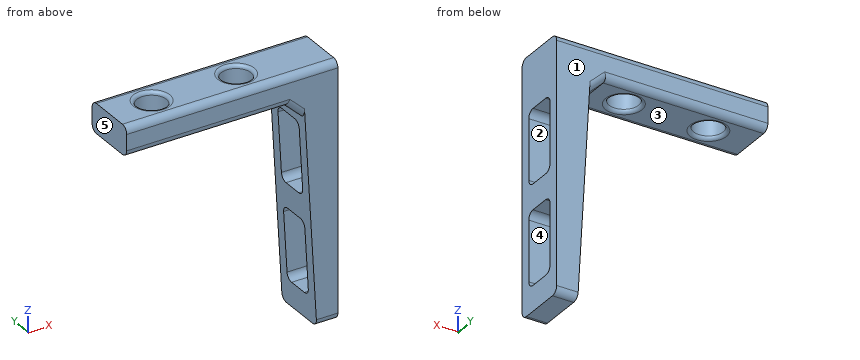
Autodesk Inventor part; units mm, degrees
ref_plane "YZ Plane" through (0, 0, 0) normal (1, 0, 0) x (0, 1, 0)
ref_plane "XZ Plane" through (0, 0, 0) normal (0, 1, 0) x (-1, 0, 0)
ref_plane "XY Plane" through (0, 0, 0) normal (0, 0, 1) x (1, 0, 0)
sketch "Szkic1" plane through (0, 0, 0) normal (0, 1, 0) x (-1, 0, 0)
  line L0 (0, 0) -> (25, 0)
  line L1 (25, 0) -> (25, -3.5)
  line L2 (25, -3.5) -> (4, -3.5)
  line L3 (4, -3.5) -> (2.5, -30)
  line L4 (2.5, -30) -> (0, -30)
  line L5 (0, -30) -> (0, 0)
  dimension "d0" = 25
  dimension "d1" = 30
  dimension "d2" = 3.5
  dimension "d3" = 2.5
  dimension "d4" = 4
extrude "Wyciągnięcie proste1" add sketch "Szkic1" along normal blind 6.5
sketch "Szkic2" plane through (0, 0, 0) normal (1, 0, 0) x (0, 0, -1)
  line L0 (0, 0) -> (30, 0)
  line L1 (30, 0) -> (30, 6.5)
  line L2 (0, 6.5) -> (30, 6.5)
  line L3 (0, 0) -> (0, 6.5)
  line L4 (30, 3.25) -> (0, 3.25) construction
  line L5 (18.25, 5.25) -> (27, 5.25)
  line L6 (27, 5.25) -> (27, 1.25)
  line L7 (27, 1.25) -> (18.25, 1.25)
  line L8 (18.25, 1.25) -> (18.25, 5.25)
  line L9 (18.25, 5.25) -> (27, 1.25) construction
  line L10 (27, 5.25) -> (18.25, 1.25) construction
  line L11 (6.5, 5.25) -> (15.25, 5.25)
  line L12 (15.25, 5.25) -> (15.25, 1.25)
  line L13 (15.25, 1.25) -> (6.5, 1.25)
  line L14 (6.5, 1.25) -> (6.5, 5.25)
  line L15 (6.5, 5.25) -> (15.25, 1.25) construction
  line L16 (15.25, 5.25) -> (6.5, 1.25) construction
  line L17 (3.5, 0) -> (3.5, 6.5)
  point P0 (22.625, 3.25)
  point P1 (10.875, 3.25)
  dimension "d7" = 26.5
  dimension "d8" = 3
  dimension "d9" = 3
  dimension "d10" = 3
  dimension "d11" = 4
extrude "Wyciągnięcie proste2" cut sketch "Szkic2" against normal up to surface contours L5 L6 L7 L8 | L11 L12 L13 L14 surface through (-2.5, 0, -30) normal (-0.9984018, 0, -0.0565133)
sketch "Szkic3" plane through (-25, 0, 0) normal (0, 0, 1) x (1, 0, 0)
  line L0 (0, 0) -> (25, 0)
  line L1 (25, 0) -> (25, 6.5)
  line L2 (0, 6.5) -> (25, 6.5) construction
  line L3 (0, 0) -> (0, 6.5)
  line L4 (0, 3.25) -> (25, 3.25) construction
  circle A0 centre (15, 3.25) radius 1.75
  circle A1 centre (5, 3.25) radius 1.75
  dimension "d14" = 3.5
  dimension "d15" = 10
  dimension "d16" = 10
extrude "Wyciągnięcie proste3" cut sketch "Szkic3" against normal up to surface (3.5 mm away)
chamfer "Faza1" distance 2 angle 45 1 edges at (-4, 3.25, -3.5)
fillet "Zaokrąglenie1" radius 0.8 16 edges at (-1.25, 6.5, -30) (-1.25, 0, -30) (-12.5, 6.5, 0) (-12.5, 0, 0) (-15.5, 0, -3.5) (-15.5, 6.5, -3.5) (-4.9435, 6.5, -4.4984) (-4.9435, 0, -4.4984) (-1.3349, 5.25, -27) (-1.5825, 5.25, -18.25) (-1.3349, 1.25, -27) (-1.5825, 1.25, -18.25) (-1.6675, 5.25, -15.25) (-1.6675, 1.25, -15.25) (-1.9151, 1.25, -6.5) (-1.9151, 5.25, -6.5)
fillet "Zaokrąglenie2" radius 0.4 4 edges at (-11.75, 3.25, -3.5) (-21.75, 3.25, -3.5) (-11.75, 3.25, 0) (-21.75, 3.25, 0)
equation "\"d9\" = d8"
properties part number "noga1"
Input: part model. Units: mm. Frame: model coordinates. Face numbers are marked on the shaded views. A direction names the side the tool comes from. Give positions to 0.01 mm unless a question says otherwise; leave off trailing zeros. Write each loop counter-clockwise with the first axis right and the second up, starting at its lowest first coordinate (ties: lowest second). Pieces come first, ordered by that corner, then holes. Notation, with made-up numbers: M -9.5,-3 L 23.5,-3 A20 cw 23.5,25 Z; hole C -17,-20 d7. An arc over 180 degrees is marked long. Use one line per item in the form item = value.
1. First-contact query: P1, Ø3, axis at y = 1.5, z = -20, coming from the -X side; P2, Ø1, axis at x = -21.5, y = 5.5, coming from the +Z side; P3, Ø2, axis at x = -19.5, y = 4, coming from the -Z side. Flat tips, straight axial feed; report the tip coordinate or a pass-through.
Outcome:
P1 = -3.15
P2 = 0
P3 = -3.41
2. Mould query, pull axis Z, two halves, no side actions, for the marked faces 3, 4 and 5. Classes: released by +Z, released by -Z, zero draft, split by the parting line, or undercut.
Outcome:
face_3 = released by -Z
face_4 = undercut
face_5 = zero draft
3. Cut plane A-A on x = -20. Return loops of the section in (y, z).
Outcome:
outline = M 0,-2.7 A0.8 ccw 0.8,-3.5 L 1.1,-3.5 A0.4 ccw 1.5,-3.1 L 1.5,-0.4 A0.4 ccw 1.1,0 L 0.8,0 A0.8 ccw 0,-0.8 Z; M 5,-3.1 A0.4 ccw 5.4,-3.5 L 5.7,-3.5 A0.8 ccw 6.5,-2.7 L 6.5,-0.8 A0.8 ccw 5.7,0 L 5.4,0 A0.4 ccw 5,-0.4 Z
4. Reachability of the marked faces 1 and 2 from +Z, -Z, +X, -X, +Y, -Y: full face, straight path, thin tool, end or side. Return the list, or none.
Outcome:
face_1 = +Z, -Z, +X, -X, +Y
face_2 = +X, -X
5. Ray query, L1, parallel to Z at x = -2, y = 3.5; L2, parallel to Y at x = -20, z = -2.1; L3, parallel to Z at x = -3, y = 2. Return the intervals inside material, ascending.
Outcome:
L1 = -30 to -27, -18.25 to -15.25, -6.5 to 0
L2 = 0 to 1.5, 5 to 6.5
L3 = -18.25 to -15.25, -6.5 to 0
6. Cut plane C-C on x = -2. Return loops of the section in (y, z).
Outcome:
outline = M 0,-29.2 A0.8 ccw 0.8,-30 L 5.7,-30 A0.8 ccw 6.5,-29.2 L 6.5,-0.8 A0.8 ccw 5.7,0 L 0.8,0 A0.8 ccw 0,-0.8 Z; hole M 1.25,-26.2 A0.8 ccw 2.05,-27 L 4.45,-27 A0.8 ccw 5.25,-26.2 L 5.25,-19.05 A0.8 ccw 4.45,-18.25 L 2.05,-18.25 A0.8 ccw 1.25,-19.05 Z; hole M 1.25,-14.45 A0.8 ccw 2.05,-15.25 L 4.45,-15.25 A0.8 ccw 5.25,-14.45 L 5.25,-7.3 A0.8 ccw 4.45,-6.5 L 2.05,-6.5 A0.8 ccw 1.25,-7.3 Z
7. Cut plane B-B on y = 3.25. State how many separate pieces and enclosed holes the cut face has, and give its area (3 significant figures).
Outcome:
separate_pieces = 5
enclosed_holes = 0
area = 94.0 mm²
8. Cut plane D-D on z = -13.5. Return loops of the section in (x, y), and give its area (3 significant figures).
Outcome:
outline = M -3.43,0 L 0,0 L 0,1.25 L -3.43,1.25 Z; M -3.43,5.25 L 0,5.25 L 0,6.5 L -3.43,6.5 Z
area = 8.58 mm²
